Design review of the part built by this model. Coordinates are the model's own, in mm. A direction names the side the tool comes from. Coordinates: 2 decimals unless noted, no trailing zeros. Write each loop counter-clockwise with the first axis right and the second up, starting at its lowest first coordinate (ties: lowest second). Pieces come first, ordered by that corner, then holes. Notation, with made-up numbers: (66.25, 37.5) - (92.25, 37.5) arc R29 ccw to (92.25, 75.5) - close; hole circle Ø2 at (23.5, 87). An arc over 180 degrees is marked (long way). Answer as CSV lines item,"result". Start each with the question number.
Q1. We need section D-D (y = 0). Write out the cut boundary in (x, z) (3 decimals).
Q2. We need section C-C (z = 1.75). Write out the cut boundary in (x, y) (3 decimals).
Q3. We need section A-A (y = 4.25). Write out the cut boundary in (x, z).
Q4. We need section B-B (x = -44.45). Write out the cut boundary in (y, z) (3 decimals).
Q5. For line 1 along X through (y, z) = (-2.25, 6); line 2 along X through (y, z) = (-2.5, 7.5); line 3 along Y through (x, z) = (-7, 2.25), list the stretches that pass through material, from the lowest coordinate up. Write a range as [from, to].
Q6. Mouldability with a two-part tool opening along Y and no side actions: class faces 1 (the face through (14.354, -9.061, 6.439)), 2 (the face through (-41.42, 0.95, 6.39)), 3 (the face through (-38.1, 0, 11)) as pulls with the +Y half, pulls with the -Y half, needs draft (parallel to the pull), parting line crosses it, or undercut.
Q7. Clearance check with flat-ended pins moving along their axes: pin 1 (2 mm diameter, centred on y = -10, z = 5.5, fed in from -X); pin 2 (8.5 mm diameter, centred on x = -44.45, y = 0, fed in from +Z); pin 3 (6.5 mm diameter, centred on x = -43, y = -2, fed in from -Z); pin 4 (10 mm diameter, centred on x = 31.5, y = 4, fed in from -Z). State where each tip first meets the part, or that it passes through.
Q8. Machinability: for faces 4 (the face through (35, -6.35, 6)), 5 (the face through (-25, -6.35, 6)), 6 (the face through (-43, 3, 9.398)), 7 (the face through (-50.8, 4, 6)), 8 (the face through (-38.1, 0, 2)), which of the approach directions +Z, -Z, +X, -X, +Y, -Y give a long, thin tool a straight path to every point of the face, cutting with its end or side? Answer none if there is none.
Autodesk Inventor part; units mm, degrees
ref_plane "YZ Plane" through (0, 0, 0) normal (1, 0, 0) x (0, 1, 0)
ref_plane "XZ Plane" through (0, 0, 0) normal (0, 1, 0) x (-1, 0, 0)
ref_plane "XY Plane" through (0, 0, 0) normal (0, 0, 1) x (1, 0, 0)
sketch "Sketch1" plane through (0, 0, 0) normal (0, 0, 1) x (1, 0, 0)
  line L0 (-50.8, -6.35) -> (50.8, -6.35)
  line L1 (50.8, -6.35) -> (50.8, 6.35)
  line L2 (50.8, 6.35) -> (-50.8, 6.35)
  line L3 (-50.8, 6.35) -> (-50.8, -6.35)
  line L4 (-50.8, -6.35) -> (50.8, 6.35) construction
  line L5 (50.8, -6.35) -> (-50.8, 6.35) construction
  point P0 (0, 0)
  dimension "d0" = 101.6
  dimension "d1" = 12.7
extrude "Extrusion1" add sketch "Sketch1" along normal blind 12.7
fillet "Fillet1" radius 7.62 1 edges at (-50.8, -6.35, 6.35)
sketch "Sketch2" plane through (0, 0, 12.7) normal (0, 0, 1) x (1, 0, 0)
  circle A0 centre (-44.45, 0) radius 3.175
  line L0 (-50.8, 6.35) -> (-50.8, 1.27)
  line L1 (50.8, 6.35) -> (-50.8, 6.35)
  point P0 (0, 0)
  dimension "d5" = 6.35
  dimension "d6" = 6.35
  dimension "d7" = 6.35
extrude "Extrusion2" cut sketch "Sketch2" against normal blind 12.7
sketch "Sketch3" plane through (0, 0, 12.7) normal (0, 0, 1) x (1, 0, 0)
  line L0 (-43.18, -6.35) -> (50.8, -6.35)
  circle A0 centre (6.35, -6.35) radius 6.35
  line L1 (-6.35, -6.35) -> (3.175, -11.8493)
  line L2 (19.05, -6.35) -> (9.525, -11.8493)
  line L3 (-50.8, 6.35) -> (-50.8, 1.27)
  point P0 (0, 0)
  dimension "d10" = 12.7
  dimension "d11" = 12.7
  dimension "d12" = 12.7
  dimension "d15" = 57.15
extrude "Extrusion3" add sketch "Sketch3" against normal blind 12.7 contours A0 L0 | L0 L2 A0 | A0 L1 L0 picked at (4.9799, -8.3631)
sketch "Sketch4" plane through (-50.8, 6.35, 0) normal (0, 1, 0) x (1, 0, 0)
  line L0 (7.62, -12.7) -> (0, -12.7)
  line L1 (0, -12.7) -> (12.7, -12.7)
  line L2 (12.7, -12.7) -> (12.7, -9.398)
  line L3 (12.7, -9.398) -> (0, -9.398)
  line L4 (0, -9.398) -> (0, -12.7)
  line L5 (0, 0) -> (12.7, 0)
  line L6 (12.7, 0) -> (12.7, -3.302)
  line L7 (12.7, -3.302) -> (0, -3.302)
  line L8 (0, -3.302) -> (0, 0)
  line L9 (101.6, 0) -> (0, 0)
  point P0 (50.8, 0)
  dimension "d16" = 12.7
  dimension "d17" = 3.302
  dimension "d21" = 3.302
extrude "Extrusion4" cut sketch "Sketch4" against normal blind 12.7
properties part number "Press_Upper_Arm"
Results list:
1,outline,"(-50.693, 3.302) - (-47.625, 3.302) - (-47.625, 9.398) - (-50.693, 9.398) - close; (-41.275, 3.302) - (-38.1, 3.302) - (-38.1, 0) - (50.8, 0) - (50.8, 12.7) - (-38.1, 12.7) - (-38.1, 9.398) - (-41.275, 9.398) - close"
2,outline,"(-38.1, -6.35) - (-6.35, -6.35) - (3.175, -11.849) arc R6.35 ccw to (9.525, -11.849) - (19.05, -6.35) - (50.8, -6.35) - (50.8, 6.35) - (-38.1, 6.35) - close"
3,outline,"(-50.8, 3.3) - (-38.1, 3.3) - (-38.1, 0) - (50.8, 0) - (50.8, 12.7) - (-38.1, 12.7) - (-38.1, 9.4) - (-50.8, 9.4) - close"
4,outline,"(-6.243, 3.302) - (-3.175, 3.302) - (-3.175, 9.398) - (-6.243, 9.398) - close; (3.175, 3.302) - (6.35, 3.302) - (6.35, 9.398) - (3.175, 9.398) - close"
5,line 1,"x = [-49.94, -46.69], [-42.21, 50.8]"
5,line 2,"x = [-49.8, -46.41], [-42.49, 50.8]"
5,line 3,"y = [-6.35, 6.35]"
6,face 1,"pulls with the -Y half"
6,face 2,"undercut"
6,face 3,"needs draft"
7,pin 1,"stops at x = -1.76"
7,pin 2,"stops at z = 9.4"
7,pin 3,"stops at z = 3.3"
7,pin 4,"stops at z = 0"
8,face 4,"+Z, -Z, +X, -Y"
8,face 5,"+Z, -Z, -X, -Y"
8,face 6,"+Z, -X, +Y, -Y"
8,face 7,"+Z, -Z, -X, +Y, -Y"
8,face 8,"-Z, -X, +Y, -Y"
